Verification items for this drawing (mm, ordinates from the low corner). A direction names the side the tool comes from. Round coordinates to 2 decimals unless told otherwise and drop trailing zeros. Loops run counter-clockwise (first coordinate to the right, second up) from the corner with the lowest first, then second, coordinate; pieces in that order, holes last. Notation, with made-up numbers: (44.25, 25) -> (59.25, 25) arc R19 ccw to (59.25, 46) -> close; hole circle Ø11 at (14.5, -21). An arc over 180 degrees is marked (long way). One line per item, written item: value. Start each with the question number.
1. Set-up check for the marked faces 1 and 2: record each of +Z, -Z, +X, -X, +Y, -Y from which the full face is reachable in a straight line by a thin tool's end or side.
2. Cross-section at A-A on x = 3. Record the cut outline in (y, z).
3. Cross-section at D-D on x = 5.55. Record the cut outline in (y, z).
4. Cross-section at C-C on z = 4.5. Record the cut outline in (x, y).
5. Go/stop test with flat-tipped pins: pin 1 (2 mm diameter, centred on y = 4, z = 2.5, fed in from +X); pin 2 (2 mm diameter, centred on y = 5, z = 2, fed in from -X); pin 3 (2 mm diameter, centred on y = 2, z = 2.5, fed in from -X). Record where each tip stops, or that it passes through.
6. Material ranges on L1, parallel to Z at x = 3.6, y = 0.35; L2, parallel to X at y = 3.05, z = 3.5; L3, parallel to Y at x = 2.9, z = 0.5, recorded low to high.
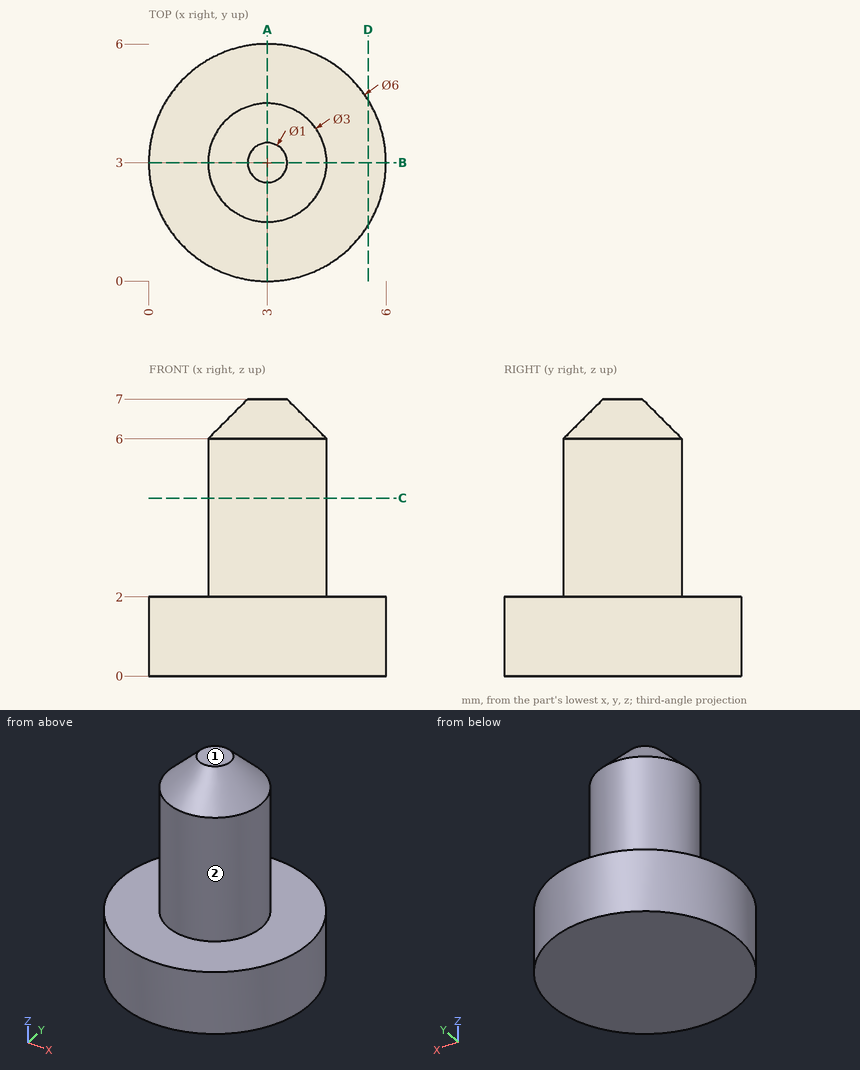
Taken from the geometry:
1. face 1: +Z, +X, -X, +Y, -Y
1. face 2: +Z
2. outline: (0, 0) -> (6, 0) -> (6, 2) -> (4.5, 2) -> (4.5, 6) -> (3.5, 7) -> (2.5, 7) -> (1.5, 6) -> (1.5, 2) -> (0, 2) -> close
3. outline: (1.42, 0) -> (4.58, 0) -> (4.58, 2) -> (1.42, 2) -> close
4. outline: circle Ø3 at (3, 3)
5. pin 1: stops at x = 6
5. pin 2: stops at x = 0.17
5. pin 3: stops at x = 0
6. L1: z = 0 to 2
6. L2: x = 1.5 to 4.5
6. L3: y = 0 to 6
